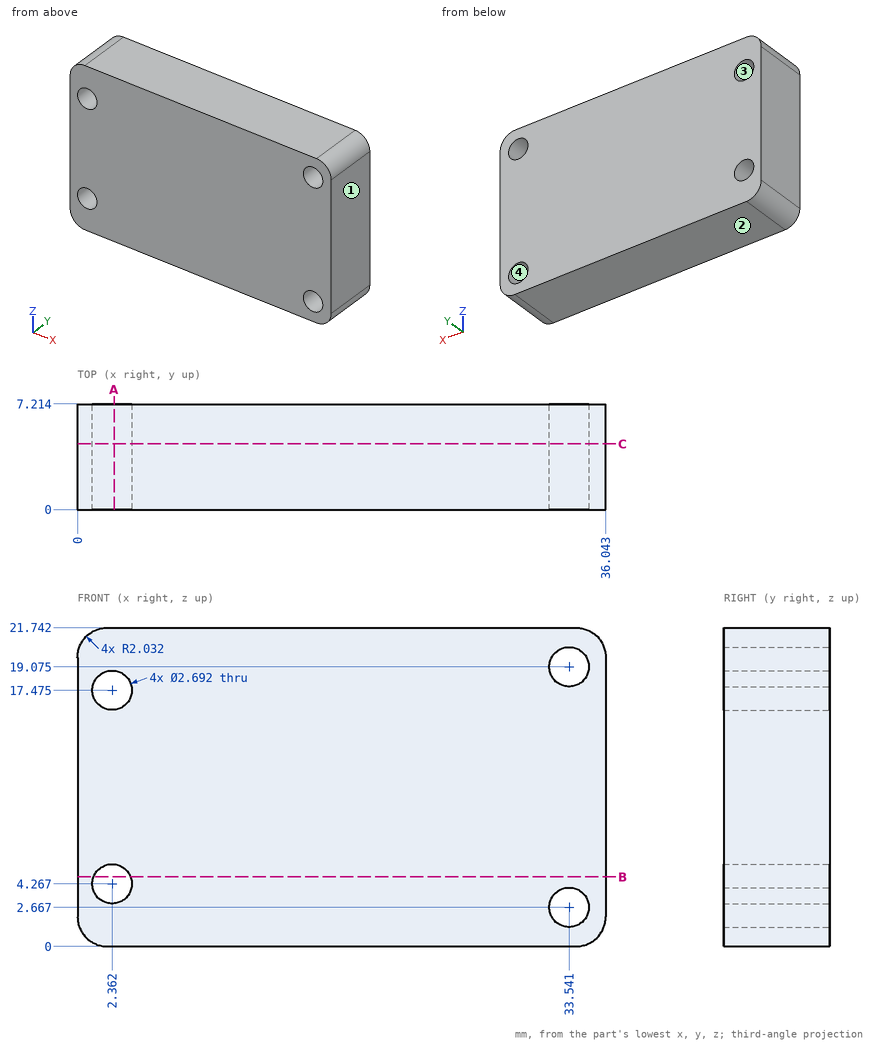
Source: three-view drawing plus pictorial views. Frame: mm from the lowest corner of the part. Coordinates: 2 decimals unless noted, no trailing zeros. Loops run counter-clockwise (first coordinate to the right, second up) from the corner with the lowest first, then second, coordinate; pieces in that order, holes last. Notation, with made-up numbers: (-10.75, 14.5) -> (29.25, 14.5) arc R27 ccw to (29.25, 40.5) -> close; hole circle Ø4 at (-37, 31). An arc over 180 degrees is marked (long way). Write each question's results on one line, items separated by ' | '. Start each with the question number.
Q1. Section A-A, the plane x = 2.5. Return the cut outline in (y, z) (1 decimal).
Q2. Ray query, line 1 (Z direction, x = 33.5, y = 5); line 2 (X direction, y = 6.5, z = 18.5) (1 decimal); line 3 (X direction, y = 3.75, z = 4.5). Return the intervals inside material, ascending. Write a range as from..to.
Q3. Pull-direction query (Z, two-part tool) for the marked faces 1, 2, 3 and 4; classes: released by +Z, released by -Z, zero draft, split by the parting line, or undercut.
Q4. Section C-C, the plane y = 4.5. Return the cut outline in (x, z) (1 decimal).
Q5. Section B-B, the plane z = 4.75. Return the cut outline in (x, y) (1 decimal), plus the area to 3 significant figures.
Found:
1) outline: (0, 0) -> (7.2, 0) -> (7.2, 2.9) -> (0, 2.9) -> close; (0, 5.6) -> (7.2, 5.6) -> (7.2, 16.1) -> (0, 16.1) -> close; (0, 18.8) -> (7.2, 18.8) -> (7.2, 21.7) -> (0, 21.7) -> close
2) line 1: 0..1.32, 4.01..17.73, 20.42..21.74 | line 2: 0..1.5, 3.2..32.3, 34.8..36 | line 3: 0..1.04, 3.69..36.04
3) face 1: zero draft | face 2: released by -Z | face 3: undercut | face 4: undercut
4) outline: (0, 2) arc R2 ccw to (2, 0) -> (34, 0) arc R2 ccw to (36, 2) -> (36, 19.7) arc R2 ccw to (34, 21.7) -> (2, 21.7) arc R2 ccw to (0, 19.7) -> close; hole circle Ø2.7 at (2.4, 4.3); hole circle Ø2.7 at (2.4, 17.5); hole circle Ø2.7 at (33.5, 2.7); hole circle Ø2.7 at (33.5, 19.1)
5) outline: (0, 0) -> (1.1, 0) -> (1.1, 7.2) -> (0, 7.2) -> close; (3.6, 0) -> (36, 0) -> (36, 7.2) -> (3.6, 7.2) -> close | area: 242 mm2
